Source: three-view drawing plus pictorial views. Frame: mm from the lowest corner of the part. Round coordinates to 2 decimals unless told otherwise and drop trailing zeros. Order: outer loops, then holes, each group sorted by start corner. A loop starts at its lowest first (then second) coordinate and runs counter-clockwise, first axis right, second up. Notation, with made-up numbers: (81.25, 25) -> (110.25, 25) arc R17 ccw to (110.25, 56) -> close; hole circle Ø11 at (3.5, 7.5). An arc over 180 degrees is marked (long way). Answer as CSV lines item,"result". Start each with the question number.
1) Section query C-C, the plane z = 25.5. Output: boundary loops of the cut face in (x, y) (3 decimals).
2) Section query A-A, the plane x = 35. Output: boundary loops of the cut face in (y, z) (3 decimals), and give its area (3 significant figures).
3) Section query B-B, the plane y = 8.5. Output: boundary loops of the cut face in (x, z) (3 decimals), and give its area (3 significant figures).
4) First-contact query: P1, Ø1, axis at y = 6.5, z = 1.5, coming from the -X side (3 decimals); P2, Ø4, axis at y = 11, z = 31.5, coming from the -X side; P3, Ø4, axis at x = 21, z = 43.5, coming from the -Y side; P4, Ø1, axis at x = 13, y = 2, coming from the +Z side (3 decimals). Flat tips, straight axial feed; report the tip coordinate or a pass-through.
5) Line query: L1, parallel to Y at x = 55.5, z = 168.5 (3 decimals); L2, parallel to Z at x = 66, y = 7.5 (3 decimals). Output: solid intervals per line, ascending.
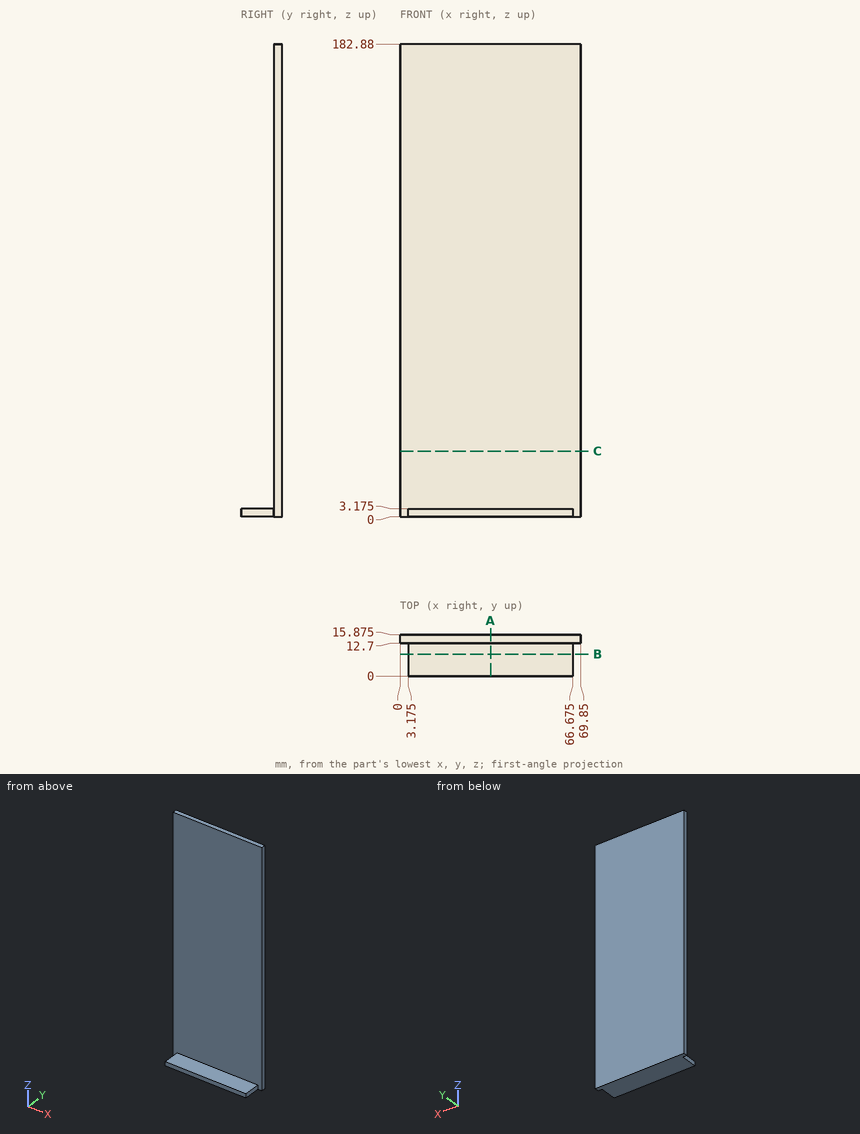
Findings:
1,outline,"(0, 12.7) -> (69.85, 12.7) -> (69.85, 15.875) -> (0, 15.875) -> close"
2,outline,"(0, 0) -> (15.875, 0) -> (15.875, 182.88) -> (12.7, 182.88) -> (12.7, 3.175) -> (0, 3.175) -> close"
2,area,"621 mm^2"
3,outline,"(3.175, 0) -> (66.675, 0) -> (66.675, 3.175) -> (3.175, 3.175) -> close"
3,area,"202 mm^2"
4,P1,"stops at x = 3.175"
4,P2,"stops at x = 0"
4,P3,"stops at y = 12.7"
4,P4,"stops at z = 3.175"
5,L1,"y = 12.7 to 15.875"
5,L2,"z = 0 to 3.175"
